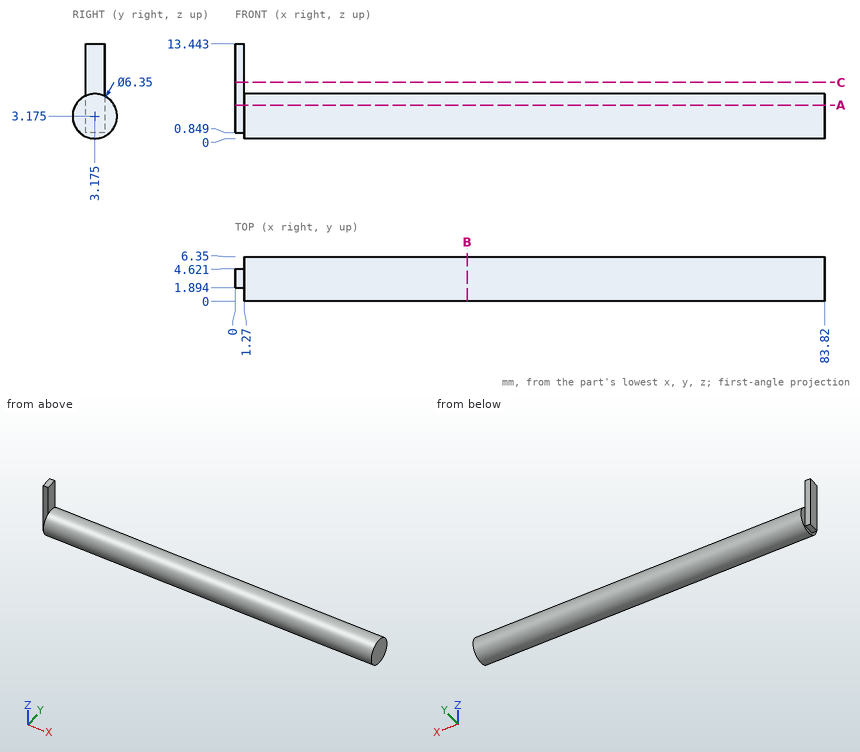
Answer from the drawing. Dimensions are ordinates in mm from the lowest x, y and z of the part. Give positions to 0.01 mm unless a question says otherwise; leave off trailing zeros. Write each loop counter-clockwise with the first axis right and the second up, starting at its lowest first coordinate (ties: lowest second). Pieces come first, ordered by that corner, then holes. Notation, with made-up numbers: (-39.75, 85) - (-10.75, 85) arc R15 cw to (-10.75, 92) - close; hole circle Ø6 at (34, 13.5). An arc over 180 degrees is marked (long way). Answer in a Markdown table with one row per item. Add a question column.
Item 1: Section B-B, the plane x = 33 is taken. Write down the section's boundary in (y, z) (3 decimals).
Item 2: Section A-A, the plane z = 4.75 is taken. Write down the section's boundary in (x, y), and give its area (3 significant figures).
Item 3: Find the intervals of material crossed by L1, parallel to X at y = 3, z = 8; L2, parallel to Y at x = 37, z = 3.25; L3, parallel to Z at x = 58, y = 0.5 (1 decimal), in increasing order.
Item 4: Flat-ended cylindrical pins translate along their axes: P1, Ø2, axis at x = 27.5, y = 4.5, coming from the -Z side; P2, Ø3, axis at y = 4, z = 10.5, coming from the +X side; P3, Ø0.6, axis at x = 0.5, y = 3.5, coming from the -Z side. Find the tip coordinate at first contact, or state that the pin passes through.
Item 5: Section C-C, the plane z = 8 is taken. Write down the section's boundary in (x, y).
Recorded:
| question | item | result |
|---|---|---|
| 1 | outline | circle Ø6.35 at (3.175, 3.175) |
| 2 | outline | (0, 1.89) - (1.27, 1.89) - (1.27, 0.42) - (83.82, 0.42) - (83.82, 5.93) - (1.27, 5.93) - (1.27, 4.62) - (0, 4.62) - close |
| 2 | area | 459 mm2 |
| 3 | L1 | x = 0 to 1.27 |
| 3 | L2 | y = 0 to 6.35 |
| 3 | L3 | z = 1.5 to 4.9 |
| 4 | P1 | stops at z = 0.02 |
| 4 | P2 | stops at x = 1.27 |
| 4 | P3 | stops at z = 0.85 |
| 5 | outline | (0, 1.89) - (1.27, 1.89) - (1.27, 4.62) - (0, 4.62) - close |
